Read the model definition and answer for the solid it produces. Units are mm, in the model's axes. Face numbers are marked on the shaded views. Round coordinates to 2 decimals unless told otherwise and drop trailing zeros. Order: outer loops, then holes, each group sorted by start corner. A loop starts at its lowest first (then second) coordinate and runs counter-clockwise, first axis right, second up. Notation, with made-up numbers: (67, 45) -> (96, 45) arc R18 ccw to (96, 65) -> close; hole circle Ø2 at (33.25, -26). An arc over 180 degrees is marked (long way). Use a Markdown table: item, result. Add a question column.
1. Consider L1, parallel to X at y = 3.5, z = -42; L2, parallel to Y at x = -24, z = -45 (3 decimals); L3, parallel to Y at x = -8, z = -34. Determine where each line is inside the solid, lowest interval first. Write a range as [from, to].
2. Section D-D, the plane x = -12.5 is taken. Give the vertices of the cut face in (y, z), then the cut area to 3 significant figures.
3. Given pin 1 (2 mm diameter, centred on x = -10, z = 13.5, fed in from +Y), flat-ended and moving along its own axis, determine where the tip first touches the part or whether it passes through.
4. Section A-A, the plane x = 12 is taken. Give the vertices of the cut face in (y, z) (3 decimals).
5. Section B-B, the plane y = 8 is taken. Give the vertices of the cut face in (x, z), then the cut area to 3 significant figures.
6. The mould has two halves that part along X. Classify the marked faces 1 and 2: +X half, -X half, draft (parallel to the pull), parting line (faces both ways), or undercut.
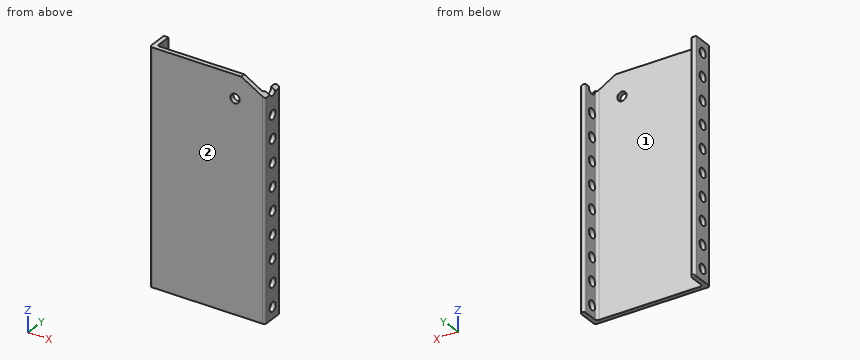
```python
from build123d import *

# Parameters (mm, degrees)
SKETCH1_W           = 50
SKETCH1_H           = 100
BOSS_EXTRUDE1_DEPTH = 2
SKETCH2_W           = 2
SKETCH2_H           = 100
BOSS_EXTRUDE2_DEPTH = 8
FILLET1_R           = 1
SKETCH3_R           = 2.005
CUT_EXTRUDE1_DEPTH  = 72.414284285
SKETCH4_R           = 2.005
CUT_EXTRUDE2_DEPTH  = 10
CUT_EXTRUDE3_DEPTH  = 57.78908359


with BuildPart() as part:
    # Sketch1 → Boss-Extrude1 (new body)
    with BuildSketch(Plane(origin=(0, 0, 0), x_dir=(1, 0, 0), z_dir=(0, 1, 0))):
        Rectangle(SKETCH1_W, SKETCH1_H)
    extrude(amount=BOSS_EXTRUDE1_DEPTH)

    # Sketch2 → Boss-Extrude2 (add)
    with BuildSketch(Plane(origin=(0, 2, 0), x_dir=(1, 0, 0), z_dir=(0, 1, 0))):
        with Locations((-24, 0)):
            Rectangle(SKETCH2_W, SKETCH2_H)
        with Locations((24, 0)):
            Rectangle(SKETCH2_W, SKETCH2_H)
    extrude(amount=BOSS_EXTRUDE2_DEPTH)

    # Fillet1
    fillet1_edges = [part.edges().sort_by_distance(p)[0] for p in [
        (-24, 10, -50),
        (-23, 10, 0),
        (-24, 10, 50),
        (-25, 10, 0),
        (25, 0, 0),
        (-25, 0, 0),
        (25, 10, 0),
        (23, 10, 0),
        (-23, 2, 0),
        (23, 2, 0),
    ]]
    fillet(fillet1_edges, radius=FILLET1_R - 0.0001)  # a hair under: the kernel refuses the full size

    # Sketch3 → Cut-Extrude1 (cut, through all)
    with BuildSketch(Plane.ZY.offset(25)):
        with Locations((-45, 5)):
            Circle(SKETCH3_R)
        with Locations((-35, 5)):
            Circle(SKETCH3_R)
        with Locations((-25, 5)):
            Circle(SKETCH3_R)
        with Locations((-15, 5)):
            Circle(SKETCH3_R)
        with Locations((-5, 5)):
            Circle(SKETCH3_R)
        with Locations((5, 5)):
            Circle(SKETCH3_R)
        with Locations((15, 5)):
            Circle(SKETCH3_R)
        with Locations((25, 5)):
            Circle(SKETCH3_R)
        with Locations((35, 5)):
            Circle(SKETCH3_R)
        with Locations((45, 5)):
            Circle(SKETCH3_R)
    extrude(amount=-CUT_EXTRUDE1_DEPTH, mode=Mode.SUBTRACT)

    # Sketch4 → Cut-Extrude2 (cut)
    with BuildSketch(Plane(origin=(0, 2, 0), x_dir=(1, 0, 0), z_dir=(0, 1, 0))):
        with Locations(Location((12, -40, 0), (0, 0, 270))):
            Circle(SKETCH4_R)
    extrude(amount=-CUT_EXTRUDE2_DEPTH, mode=Mode.SUBTRACT)

    # Sketch5 → Cut-Extrude3 (cut, through all)
    with BuildSketch(Plane.XZ):
        Polygon((25, 50), (14.68, 50), (25, 44.04), align=None)
    extrude(amount=-CUT_EXTRUDE3_DEPTH, mode=Mode.SUBTRACT)


solid = part.part
```
Verdict:
| question | item | result |
|---|---|---|
| 1 | L1 | x = [-25, -23], [23, 25] |
| 1 | L2 | y = [0, 2.995], [7.005, 10] |
| 1 | L3 | y = [0, 2] |
| 2 | outline | (0, -50) -> (2, -50) -> (2, 50) -> (0, 50) -> close |
| 2 | area | 200 mm2 |
| 3 | pin 1 | stops at y = 2 |
| 4 | outline | (0, -50) -> (2, -50) -> (2, 37.995) -> (0, 37.995) -> close; (0, 42.005) -> (2, 42.005) -> (2, 50) -> (0, 50) -> close |
| 5 | outline | (-25, -50) -> (-23, -50) -> (-23, 50) -> (-25, 50) -> close; (23, -50) -> (25, -50) -> (25, 44.04) -> (23, 45.2) -> close |
| 5 | area | 389 mm2 |
| 6 | face 1 | undercut |
| 6 | face 2 | draft |
